For this review, take the finished solid that the model builds, in its own axes (mm). A direction names the side the tool comes from. Round coordinates to 2 decimals unless told otherwise and drop trailing zeros. Write each loop counter-clockwise with the first axis right and the second up, starting at its lowest first coordinate (ties: lowest second). Pieces come first, ordered by that corner, then holes. Notation, with made-up numbers: (78, 30) -> (133, 30) arc R29 ccw to (133, 56) -> close; hole circle Ø3 at (7.5, 76). An arc over 180 degrees is marked (long way). Answer in a Markdown table with one row per item.
from build123d import *

# Parameters (mm, degrees)
F0_W     = 53
F0_H     = 53
F1_DEPTH = 60
F3_DEPTH = 4


with BuildPart() as f1:
    # F0 (on Right) → F1 (new body)
    with BuildSketch(Plane.YZ):
        with Locations((26.5, 26.5)):
            Rectangle(F0_W, F0_H)
    extrude(amount=F1_DEPTH)

    # F2 (on face) → F3 (cut)
    with BuildSketch(Plane.XY.offset(53)):
        with BuildLine():
            ThreePointArc((12, 33), (8, 37), (4, 33))
            Line((4, 33), (4, 8))
            ThreePointArc((4, 8), (5.171573, 5.171573), (8, 4))
            Line((8, 4), (33, 4))
            ThreePointArc((33, 4), (37, 8), (33, 12))
            Line((33, 12), (12, 12))
            Line((12, 12), (12, 33))
        make_face()
    extrude(amount=-F3_DEPTH, mode=Mode.SUBTRACT)


solid = f1.part
1) Mouldability with a two-part tool opening along X and no side actions: class faces 3 (the flat face through (0, 26, 27)), 4 (the flat face through (60, 26, 27)), 5 (the flat face through (30, 0, 26)), 6 (the flat face through (20, 4, 51)) as pulls with the +X half, pulls with the -X half, needs draft (parallel to the pull), parting line crosses it, or undercut.
Solved:
| item | result |
|---|---|
| face 3 | pulls with the -X half |
| face 4 | pulls with the +X half |
| face 5 | needs draft |
| face 6 | undercut |
2) Consider section A-A on y = 5.5. State the section outline as (x, z) points.
Solved:
| item | result |
|---|---|
| outline | (0, 0) -> (60, 0) -> (60, 53) -> (36.12, 53) -> (36.12, 49) -> (4.88, 49) -> (4.88, 53) -> (0, 53) -> close |
3) For line 1 (Z direction, x = 30.5, y = 5), list the stretches that pass through material, from the lowest coordinate up. Write a range as [from, to].
Solved:
| item | result |
|---|---|
| line 1 | [0, 49] |
4) For faces 1 (the flat face through (23, 12, 51)), 2 (the flat face through (30, 53, 26)), list the 3-axis set-ups (+Z, -Z, +X, -X, +Y, -Y) from which the entire face can be reached by the end or side of a thin tool; tool diameter is ignored.
Solved:
| item | result |
|---|---|
| face 1 | +Z |
| face 2 | +Z, -Z, +X, -X, +Y |
